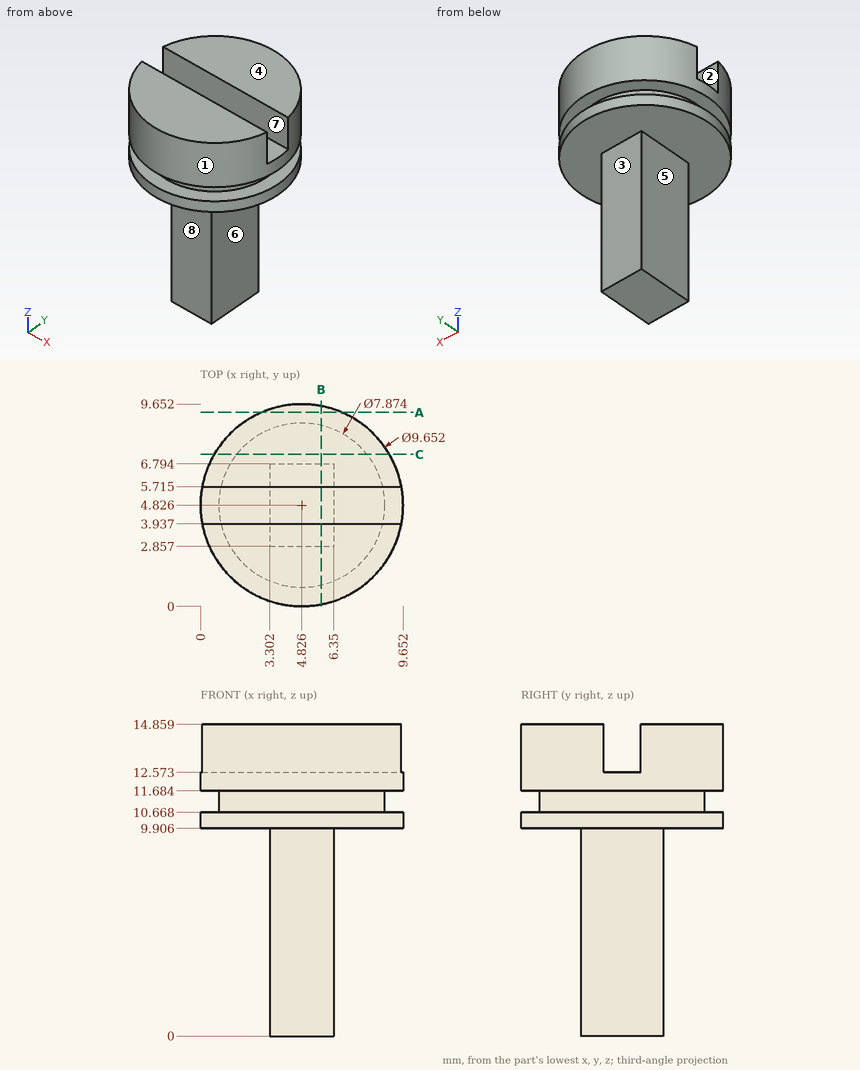
For this review, use the dimensioned drawing (mm, ordinates from the lowest corner) and the shaded views. A direction names the side the tool comes from. Give positions to 0.01 mm unless a question says otherwise; leave off trailing zeros. Order: outer loops, then holes, each group sorted by start corner. A loop starts at its lowest first (then second) coordinate and runs counter-clockwise, first axis right, second up. Notation, with made-up numbers: M -34.5,12.25 L 17.5,12.25 A30 ccw 17.5,37.25 Z; hole C 89.5,64 d6. An arc over 180 degrees is marked long. Use one line per item in the form item = value. Start each with the question number.
Item 1: For the marked faces 5, 6, 7 and 8, list the 3-axis set-ups (+Z, -Z, +X, -X, +Y, -Y) from which the entire face can be reached by the end or side of a thin tool; tool diameter is ignored.
Item 2: Insertion check: pin 1 Ø0.9 at (x, z) = (4.5, 3) entering from -Y; pin 2 Ø5 at (x, z) = (2.5, 4) entering from +Y (1 decimal); pin 3 Ø1 at (y, z) = (8.5, 3.5) entering from -X; pin 4 Ø1.8 at (x, z) = (3, 13.5) entering from +Y. Each pin has a flat end and moves straight along its axis. Give the tip position at first contact, or say it passes through.
Item 3: The part is to be moulded in two halves that separate along Y. For the marked faces 1, 2, 3 and 4, say which applies: pulls with the +Y half, pulls with the -Y half, needs draft (parallel to the pull), parting line crosses it, or undercut.
Item 4: We need section B-B on x = 5.75. Give the boundary of the cut face in (y, z) (1 decimal).
Item 5: We need section A-A on y = 9.25. Give the boundary of the cut face in (x, z) (1 decimal), plus the area to 3 significant figures.
Item 6: We need section C-C on y = 7.25. Give the boundary of the cut face in (x, z) (1 decimal).
Item 7: To check wall thickness, follow line 1 along Z through (x, y) = (8, 2) (1 decimal); line 2 along X through (y, z) = (4.5, 3.75); line 3 along Z through (x, y) = (2.25, 2.5) (1 decimal). State the ranges of each line that lie inside material, in increasing order. Write a range as from..to.
Completed:
q1.face_5 = -Z, -X, +Y, -Y
q1.face_6 = -Z, +X, +Y, -Y
q1.face_7 = +Z, +X, -X
q1.face_8 = -Z, +X, -X, -Y
q2.pin_1 = 2.86
q2.pin_2 = 6.8
q2.pin_3 = through
q2.pin_4 = 9.56
q3.face_1 = parting line crosses it
q3.face_2 = undercut
q3.face_3 = pulls with the +Y half
q3.face_4 = needs draft
q4.outline = M 0.1,9.9 L 2.9,9.9 L 2.9,0 L 6.8,0 L 6.8,9.9 L 9.6,9.9 L 9.6,10.7 L 8.7,10.7 L 8.7,11.7 L 9.6,11.7 L 9.6,14.9 L 5.7,14.9 L 5.7,12.6 L 3.9,12.6 L 3.9,14.9 L 0.1,14.9 L 0.1,11.7 L 1,11.7 L 1,10.7 L 0.1,10.7 Z
q5.outline = M 2.9,9.9 L 6.8,9.9 L 6.8,10.7 L 2.9,10.7 Z; M 2.9,11.7 L 6.8,11.7 L 6.8,14.9 L 2.9,14.9 Z
q5.area = 15.2 mm²
q6.outline = M 0.7,9.9 L 9,9.9 L 9,10.7 L 7.9,10.7 L 7.9,11.7 L 9,11.7 L 9,14.9 L 0.7,14.9 L 0.7,11.7 L 1.7,11.7 L 1.7,10.7 L 0.7,10.7 Z
q7.line_1 = 9.9..10.7, 11.7..14.9
q7.line_2 = 3.3..6.35
q7.line_3 = 9.9..14.9
